```python
from build123d import *

# Parameters (mm, degrees)
BOSS_EXTRUDE1_DEPTH    = 3.175
F_10_CLEARANCE_HOLE1_D = 5.1054


with BuildPart() as part:
    # Sketch1 → Boss-Extrude1 (new body)
    with BuildSketch(Plane.XY):
        with BuildLine():
            Line((0, 0), (25.4, 0))
            Line((25.4, 0), (25.4, 76.2))
            ThreePointArc((25.4, 76.2), (63.5, 114.3), (101.6, 76.2))
            Line((101.6, 76.2), (127, 76.2))
            ThreePointArc((127, 76.2), (63.5, 139.7), (0, 76.2))
            Line((0, 76.2), (0, 0))
        make_face()
    extrude(amount=BOSS_EXTRUDE1_DEPTH)

    # #10 Clearance Hole1 (through all)
    with Locations(Plane(origin=(0, 0, 0), x_dir=(-1, 0, 0), z_dir=(0, 0, -1))):
        with Locations((-12.7, 25.4), (-12.7, 50.8)):
            Hole(F_10_CLEARANCE_HOLE1_D / 2)


solid = part.part
```
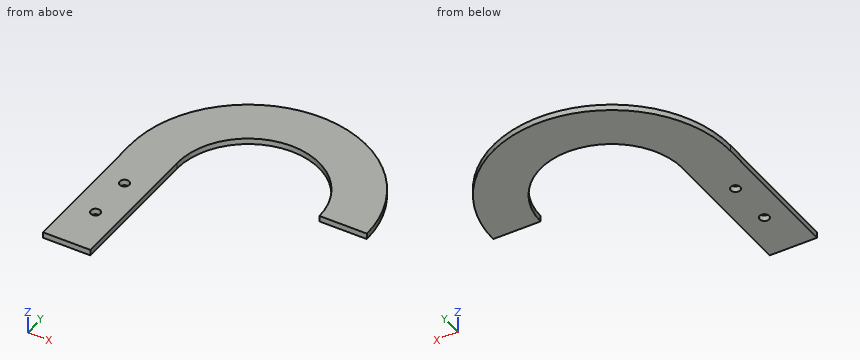
The listing builds one solid part. Answer for the finished solid, in the listing's coordinates (mm). Coordinates: 2 decimals unless noted, no trailing zeros. Order: outer loops, then holes, each group sorted by start corner. A loop starts at its lowest first (then second) coordinate and runs counter-clockwise, first axis right, second up. Notation, with made-up numbers: M 23.25,73 L 60.25,73 A6 cw 60.25,84 Z; hole C 64.25,74.25 d6. An arc over 180 degrees is marked long. Answer as a JSON object with one key per item and string values. Group by question number.
1. Section A-A on x = 12.7 is taken. Write down the section's boundary in (y, z) (3 decimals), then the cut area to 3 significant figures.
2. Flat-ended cylindrical pins translate along their axes: P1, Ø4, axis at x = 12.7, y = 25.4, coming from the +Z side; P2, Ø1, axis at x = 25.5, z = 2, coming from the +Y side; P3, Ø1.5, axis at y = 86.5, z = 0.5, coming from the +X side; P4, Ø1.5, axis at y = 95, z = 2.5, coming from the -X side. Find the tip coordinate at first contact, or state that the pin passes through.
3. Section C-C on z = 2.15 is taken. Write down the section's boundary in (x, y).
4. Section D-D on x = 63.5 is taken. Write down the section's boundary in (y, z) (3 decimals), then the cut area to 3 significant figures.
5. Straight lines are drawn through the part: line 1 (Y direction, x = 12.7, z = 2.2); line 2 (X direction, y = 37.5, z = 0.35); line 3 (X direction, y = 26, z = 1.45). For each, find the intervals that lie inside material, in ascending order.
6. Section B-B on y = 50.8 is taken. Write down the section's boundary in (x, z) (3 decimals), then the cut area to 3 significant figures.
Values follow:
{
 "1": {"outline": "M 0,0 L 22.847,0 L 22.847,3.175 L 0,3.175 Z; M 27.953,0 L 48.247,0 L 48.247,3.175 L 27.953,3.175 Z; M 53.353,0 L 114.3,0 L 114.3,3.175 L 53.353,3.175 Z", "area": "330 mm2"},
 "2": {"P1": "through", "P2": "y = 127.44", "P3": "x = 126.28", "P4": "x = 2.62"},
 "3": {"outline": "M 0,0 L 25.4,0 L 25.4,76.2 A38.1 cw 101.6,76.2 L 127,76.2 A63.5 ccw 0,76.2 Z; hole C 12.7,25.4 d5.11; hole C 12.7,50.8 d5.11"},
 "4": {"outline": "M 114.3,0 L 139.7,0 L 139.7,3.175 L 114.3,3.175 Z", "area": "80.6 mm2"},
 "5": {"line 1": "0 to 22.85, 27.95 to 48.25, 53.35 to 114.3", "line 2": "0 to 25.4", "line 3": "0 to 10.22, 15.18 to 25.4"},
 "6": {"outline": "M 0,0 L 10.147,0 L 10.147,3.175 L 0,3.175 Z; M 15.253,0 L 25.4,0 L 25.4,3.175 L 15.253,3.175 Z", "area": "64.4 mm2"}
}
